Could you check a few things on this model? Use its own coordinates, in mm. Coordinates: 2 decimals unless noted, no trailing zeros. Loops run counter-clockwise (first coordinate to the right, second up) from the corner with the lowest first, then second, coordinate; pieces in that order, holes last. Notation, with made-up numbers: M 64.5,27 L 90.5,27 A20 ccw 90.5,37 Z; hole C 52,-19.5 d11. An arc over 180 degrees is marked long. Write each question's results on one line, items separated by ' | '.
```python
from build123d import *

# Parameters (mm, degrees)
BOSS_EXTRUDE1_DEPTH               = 3.175
SKETCH8_W                         = 36.346
SKETCH8_H                         = 3.175
BOSS_EXTRUDE3_DEPTH               = 3.175
SKETCH7_R                         = 2
LED_HOLE_DEPTH                    = 4.175
SKETCH10_W                        = 36.346
SKETCH10_H                        = 12.319
LOWER_PART_DEPTH                  = 3.175
CUT_EXTRUDE3_DEPTH                = 4.175
SKETCH11_W                        = 4.32
SKETCH11_H                        = 5.08
SKETCH11_W_2                      = 4.315
IR_HOLE_DEPTH                     = 4.175
SKETCH14_W                        = 24.003
SKETCH14_H                        = 37.717280076
SKETCH14_W_2                      = 22
BOSS_EXTRUDE5_DEPTH               = 3.175
SKETCH19_W                        = 3.175
SKETCH19_H                        = 1.5
BOTTOM_GROOVE_FOR_SIDE_PART_DEPTH = 3.175


with BuildPart() as part:
    # Sketch1 → Boss-Extrude1 (new body)
    with BuildSketch(Plane.XY):
        Polygon((-27.39024803, -18.912140652), (-12.39024803, -18.912140652), (-12.39024803, -33.912140652), (-1.71724803, -33.912140652), (-1.71724803, -14.863860576), (-38.06324803, -14.863860576), (-38.06324803, -33.912140652), (-27.39024803, -33.912140652), align=None)
    extrude(amount=-BOSS_EXTRUDE1_DEPTH)

    # Sketch8 → Boss-Extrude3 (add)
    with BuildSketch(Plane.XY):
        with Locations((-19.89024803, -35.499640652)):
            Rectangle(SKETCH8_W, SKETCH8_H)
        with Locations((-19.89024803, -13.276360576)):
            Rectangle(SKETCH8_W, SKETCH8_H)
    extrude(amount=-BOSS_EXTRUDE3_DEPTH)

    # Sketch7 → LED hole (cut, through all)
    with BuildSketch(Plane.XY):
        with Locations((-19.752796976, -16.027063068)):
            Circle(SKETCH7_R)
    extrude(amount=-LED_HOLE_DEPTH, mode=Mode.SUBTRACT)

    # Sketch10 → Lower part (add)
    with BuildSketch(Plane.XY):
        with Locations((-19.89024803, -43.246640652)):
            Rectangle(SKETCH10_W, SKETCH10_H)
    extrude(amount=-LOWER_PART_DEPTH)

    # Sketch12 → Cut-Extrude3 (cut, through all)
    with BuildSketch(Plane(origin=(0, 0, -3.175), x_dir=(-1, 0, 0), z_dir=(0, 0, -1))):
        Polygon((12.39024803, -33.912140652), (12.39024803, -18.912140652), (9.21524803, -18.912140652), (9.21524803, -22.092140652), (9.21524803, -30.737140652), (9.21524803, -33.912140652), align=None)
        Polygon((27.39024803, -18.912140652), (27.39024803, -33.912140652), (30.56524803, -33.912140652), (30.56524803, -30.732140652), (30.56524803, -22.087140652), (30.56524803, -18.912140652), align=None)
    extrude(amount=-CUT_EXTRUDE3_DEPTH, mode=Mode.SUBTRACT)

    # Sketch11 → IR Hole (cut, through all)
    with BuildSketch(Plane.XY):
        with Locations((-32.72524803, -27.872140652)):
            Rectangle(SKETCH11_W, SKETCH11_H)
        with Locations((-7.057813242, -27.872140652)):
            Rectangle(SKETCH11_W_2, SKETCH11_H)
    extrude(amount=-IR_HOLE_DEPTH, mode=Mode.SUBTRACT)

    # Sketch14 → Boss-Extrude5 (add)
    with BuildSketch(Plane(origin=(0, 0, -3.175), x_dir=(-1, 0, 0), z_dir=(0, 0, -1))):
        with Locations((-10.28425197, -30.547500614)):
            Rectangle(SKETCH14_W, SKETCH14_H)
        with Locations((49.06324803, -30.547500614)):
            Rectangle(SKETCH14_W_2, SKETCH14_H)
    extrude(amount=-BOSS_EXTRUDE5_DEPTH)

    # Sketch19 → bottom groove for side part (cut)
    with BuildSketch(Plane.XY):
        with Locations((-28.97774803, -34.662140652)):
            Rectangle(SKETCH19_W, SKETCH19_H)
        with Locations((-10.80274803, -34.662140652)):
            Rectangle(SKETCH19_W, SKETCH19_H)
    extrude(amount=-BOTTOM_GROOVE_FOR_SIDE_PART_DEPTH, mode=Mode.SUBTRACT)

    # Mirror1: part across plane


with BuildPart() as part_1:
    add(part.part)
    add(part.part.mirror(Plane(origin=(22.28575197, 0, 0), x_dir=(0, 0, 1), z_dir=(1, 0, 0))))


solid = part_1.part
```
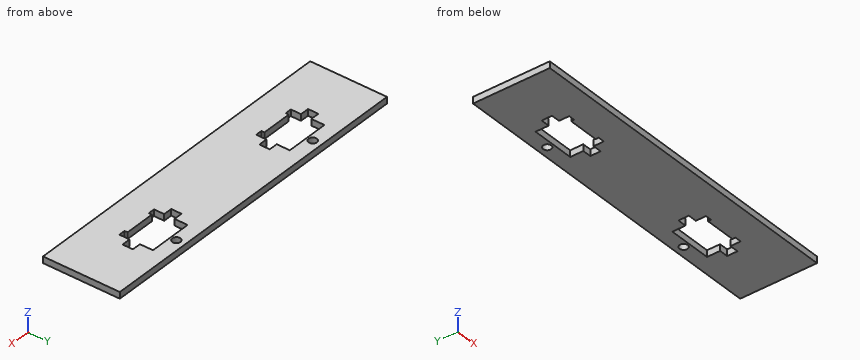
(1) Will this pin go through, and if not, where does the flat tip stop? P1, Ø8, axis at x = 64, y = -29, coming from the -Z side.
Reported:
P1: passes through
(2) Imagine slicing it at B-B, the plane z = -1.25. State how many separate pieces and enclosed holes the cut face has, and give its area (3 significant figures).
Reported:
separate pieces: 1 | enclosed holes: 4 | area: 5,440 mm2
(3) Imagine slicing it at A-A, the plane x = 68. List the corners of the cut face in (y, z) for me (3 decimals), and give its area (3 significant figures).
Reported:
outline: M -49.406,-3.175 L -33.912,-3.175 L -33.912,0 L -49.406,0 Z; M -18.912,-3.175 L -11.689,-3.175 L -11.689,0 L -18.912,0 Z | area: 72.1 mm2
(4) Please list where these lines run through material, in increasing order: probe 1 along X at (y, z) = (-21, -1.85); probe 2 along X at (y, z) = (-27, -2.65); probe 3 along Y at (x, z) = (69, -1.1). Write a range as from..to.
Reported:
probe 1: x = -60.06..-30.57, -9.22..53.79, 75.14..104.63 | probe 2: x = -60.06..-34.89, -4.9..49.47, 79.46..104.63 | probe 3: y = -49.41..-33.91, -18.91..-11.69
